from build123d import *

# Parameters (mm, degrees)
SKETCH1_W           = 0.9
SKETCH1_H           = 1.1
BOSS_EXTRUDE1_DEPTH = 14.8
CHAMFER1_SIZE       = 0.3


with BuildPart() as part:
    # Sketch1 → Boss-Extrude1 (new body)
    with BuildSketch(Plane.XY):
        with BuildLine():
            Line((1.1, -0.033079582), (0.5, -10))
            ThreePointArc((0.5, -10), (0.969051295, -10.529141647), (1.498192942, -10.060090353))
            Line((1.498192942, -10.060090353), (2.098192942, -0.093169935))
            ThreePointArc((2.098192942, -0.093169935), (0.597103418, 1.549796772), (-1, 0))
            Line((-1, 0), (-1, -12))
            ThreePointArc((-1, -12), (-0.5, -12.5), (0, -12))
            Line((0, -12), (0, 0))
            ThreePointArc((0, 0), (0.567044659, 0.550248639), (1.1, -0.033079582))
        make_face()
        with Locations((-1.45, -0.55)):
            Rectangle(SKETCH1_W, SKETCH1_H)
        with Locations((-1.45, -6.75)):
            Rectangle(SKETCH1_W, SKETCH1_H)
    extrude(amount=BOSS_EXTRUDE1_DEPTH)

    # Chamfer1
    chamfer1_edges = [part.edges().sort_by_distance(p)[0] for p in [
        (0.969051295, -10.529141647, 14.8),
        (1.798192942, -5.076630144, 14.8),
        (0.567044659, 0.550248639, 0),
        (0, -6, 0),
        (-0.5, -12.5, 0),
        (-1, -9.65, 0),
        (0.597103418, 1.549796772, 14.8),
        (0.597103418, 1.549796772, 0),
        (1.798192942, -5.076630144, 0),
        (0.969051295, -10.529141647, 0),
        (0.8, -5.016539791, 0),
        (0.8, -5.016539791, 14.8),
        (-1, -9.65, 14.8),
        (-0.5, -12.5, 14.8),
        (0, -6, 14.8),
        (0.567044659, 0.550248639, 14.8),
    ]]
    chamfer(chamfer1_edges, length=CHAMFER1_SIZE)


solid = part.part
Could you check a few things on this model? Use its own coordinates, in mm. A direction names the side the tool comes from. Coordinates: 2 decimals unless noted, no trailing zeros. Order: outer loops, then holes, each group sorted by start corner. A loop starts at its lowest first (then second) coordinate and runs counter-clockwise, first axis right, second up.
Q1. Suppose I cut it at A-A on y = -9.25. Please give me the cut outline in (x, z).
Q2. Suppose I cut it at D-D on y = -3.5. Please give me the cut outline in (x, z).
Q3. Suppose I cut it at B-B on z = 14. Please give me the cut outline in (x, y), and give its area (3 significant figures).
Q4. Please list where these lines run through material, in increasing order: L1, parallel to Y at x = -1.5, z = 8.75; L2, parallel to X at y = -10.25, z = 7.5; L3, parallel to X at y = -5.5, z = 6.75.
Q5. Which directions (+Z, -Z, +X, -X, +Y, -Y) give clear straight access to the entire face, cutting with the end or side of a thin tool? Please do faces 4 (the flat face through (-1, -4, 7)), 5 (the flat face through (0, -6, 7)), 6 (the flat face through (0.956, -4.956, 0.148)), 7 (the flat face through (0.804, -4.947, 7.301)).
Q6. Suppose I cut it at C-C on y = -11.5. Please give me the cut outline in (x, z), and give its area (3 significant figures).
Q7. Thinking about a two-plate mould opening in Y: for faces 1 (the flat face through (1.642, -5.137, 14.652)), 2 (the flat face through (-1.4, 0, 7.3)), 3 (the flat face through (-1.5, -6.2, 7.3)), which applies, released by +Y, released by -Y, zero draft, split by the parting line, or undercut?
Q8. Will these pins go through, and if not, where does the flat tip stop? pin 1 (1.5 mm diameter, centred on x = 0.5, y = -2, fed in from +Z); pin 2 (1.4 mm diameter, centred on y = -9.5, z = 6, fed in from -X).
Answer:
1. outline: (-1, 0.3) - (-0.7, 0) - (-0.3, 0) - (0, 0.3) - (0, 14.5) - (-0.3, 14.8) - (-0.7, 14.8) - (-1, 14.5) - close; (0.55, 0.3) - (0.85, 0) - (1.25, 0) - (1.55, 0.3) - (1.55, 14.5) - (1.25, 14.8) - (0.85, 14.8) - (0.55, 14.5) - close
2. outline: (-1, 0) - (-0.3, 0) - (0, 0.3) - (0, 14.5) - (-0.3, 14.8) - (-1, 14.8) - close; (0.89, 0.3) - (1.19, 0) - (1.59, 0) - (1.89, 0.3) - (1.89, 14.5) - (1.59, 14.8) - (1.19, 14.8) - (0.89, 14.5) - close
3. outline: (-1.9, -7.3) - (-1, -7.3) - (-1, -12) arc R0.5 ccw to (0, -12) - (0, 0) arc R0.55 cw (long way) to (1.1, -0.03) - (0.5, -10) arc R0.5 ccw to (1.5, -10.06) - (2.1, -0.09) arc R1.55 ccw (long way) to (-1, 0) - (-1.9, 0) - (-1.9, -1.1) - (-1, -1.1) - (-1, -6.2) - (-1.9, -6.2) - close
3. area: 28.1 mm2
4. L1: y = -7.3 to -6.2, -1.1 to 0
4. L2: x = -1 to 0, 0.55 to 1.45
4. L3: x = -1 to 0, 0.77 to 1.77
5. face 4: +Z, -Z, -X
5. face 5: +Z, -Z, -Y
5. face 6: -Z
5. face 7: +Z, -Z
6. outline: (-1, 0.3) - (-0.7, 0) - (-0.3, 0) - (0, 0.3) - (0, 14.5) - (-0.3, 14.8) - (-0.7, 14.8) - (-1, 14.5) - close
6. area: 14.6 mm2
7. face 1: released by -Y
7. face 2: released by +Y
7. face 3: undercut
8. pin 1: stops at z = 14.77
8. pin 2: stops at x = -1
